For this review, take the finished solid that the model builds, in its own axes (mm). A direction names the side the tool comes from. Coordinates: 2 decimals unless noted, no trailing zeros. Loops run counter-clockwise (first coordinate to the right, second up) from the corner with the lowest first, then second, coordinate; pieces in that order, holes last. Notation, with made-up numbers: (-36.5, 54) -> (-26.5, 54) arc R27 ccw to (-26.5, 83) -> close; hole circle Ø6 at (70.5, 78). An arc over 180 degrees is marked (long way). Use a Markdown table: item, result.
from build123d import *

# Parameters (mm, degrees)
SKETCH_R     = 4.2
PAD_DEPTH    = 3
SKETCH001_R  = 3.75
PAD001_DEPTH = 3.25
FILLET_R     = 1


with BuildPart() as part:
    # Sketch → Pad (new body)
    with BuildSketch(Plane.XY):
        Circle(SKETCH_R)
    extrude(amount=PAD_DEPTH)

    # Sketch001 (on Face3 of Pad) → Pad001 (join)
    with BuildSketch(Plane.XY.offset(3)):
        Circle(SKETCH001_R)
    extrude(amount=PAD001_DEPTH)

    # Fillet
    fillet_edges = [part.edges().sort_by_distance(p)[0] for p in [
        (-3.75, 0, 6.25),
    ]]
    fillet(fillet_edges, radius=FILLET_R)


solid = part.part
(1) Take a section at D-D on z = 1. Write out the cut boundary in (x, y).
Found:
| item | result |
|---|---|
| outline | circle Ø8.4 at (0, 0) |
(2) For faces 1 (the face through (0, 0, 0)), 2 (the face through (-3.746, 0.165, 4.109)), list the 3-axis set-ups (+Z, -Z, +X, -X, +Y, -Y) from which the entire face can be reached by the end or side of a thin tool; tool diameter is ignored.
Found:
| item | result |
|---|---|
| face 1 | -Z, +X, -X, +Y, -Y |
| face 2 | +Z |
(3) Take a section at A-A on y = 0. Write out the cut boundary in (x, z), plus the area to 3 significant figures.
Found:
| item | result |
|---|---|
| outline | (-4.2, 0) -> (4.2, 0) -> (4.2, 3) -> (3.75, 3) -> (3.75, 5.25) arc R1 ccw to (2.75, 6.25) -> (-2.75, 6.25) arc R1 ccw to (-3.75, 5.25) -> (-3.75, 3) -> (-4.2, 3) -> close |
| area | 49.1 mm^2 |
(4) For line 1 along Y through (x, z) = (0, 4.5); line 2 along Z through (x, y) = (-2, 3.25); line 3 along X through (y, z) = (1.5, 3.5), list the stretches that pass through material, from the lowest coordinate up.
Found:
| item | result |
|---|---|
| line 1 | y = -3.75 to 3.75 |
| line 2 | z = 0 to 3 |
| line 3 | x = -3.44 to 3.44 |
(5) For pin 1 Ø1 at (x, y) = (-0.5, 0.5) entering from -Z; pin 2 Ø2 at (x, z) = (-0.5, 5) entering from -Y; pin 3 Ø1 at (y, z) = (2.5, 1) entering from +X, all flat-tipped, find the tip position at first contact; note any pin that passes through.
Found:
| item | result |
|---|---|
| pin 1 | stops at z = 0 |
| pin 2 | stops at y = -3.75 |
| pin 3 | stops at x = 3.69 |
(6) Take a section at C-C on z = 4. Write out the cut boundary in (x, y).
Found:
| item | result |
|---|---|
| outline | circle Ø7.5 at (0, 0) |
